from build123d import *

# Parameters (mm, degrees)
SKETCH1_R           = 3
BOSS_EXTRUDE1_DEPTH = 4.3
SKETCH2_R           = 4.92
SKETCH2_R_2         = 3
BOSS_EXTRUDE2_DEPTH = 1.5
FILLET1_R           = 0.6
CHAMFER1_SIZE       = 0.3


with BuildPart() as part:
    # Sketch1 → Boss-Extrude1 (new body)
    with BuildSketch(Plane.XY):
        Polygon((-2.840563324, 4.92), (2.840563324, 4.92), (5.681126649, 0), (2.840563324, -4.92), (-2.840563324, -4.92), (-5.681126649, 0), align=None)
        Circle(SKETCH1_R, mode=Mode.SUBTRACT)
    extrude(amount=BOSS_EXTRUDE1_DEPTH)

    # Sketch2 → Boss-Extrude2 (add)
    with BuildSketch(Plane.XY.offset(4.3)):
        Circle(SKETCH2_R)
        Circle(SKETCH2_R_2, mode=Mode.SUBTRACT)
    extrude(amount=BOSS_EXTRUDE2_DEPTH)

    # Fillet1
    fillet1_edges = [part.edges().sort_by_distance(p)[0] for p in [
        (-4.92, 0, 5.8),
    ]]
    fillet(fillet1_edges, radius=FILLET1_R)

    # Sketch3 → Cut-Revolve1 (revolve, cut)
    with BuildSketch(Plane(origin=(0, 0, 0), x_dir=(0, 0, -1), z_dir=(1, 0, 0))):
        Polygon((-4.3, 4.92), (-3.475971619, 5.575), (-0.824028381, 5.575), (0, 4.92), (0, 6.412884747), (-4.3, 6.412884747), align=None)
    revolve(axis=Axis((0, 0, 0), (0, 0, -1)), mode=Mode.SUBTRACT)

    # Chamfer1
    chamfer1_edges = [part.edges().sort_by_distance(p)[0] for p in [
        (-3, 0, 0),
    ]]
    chamfer(chamfer1_edges, length=CHAMFER1_SIZE)


solid = part.part
The listing builds one solid part. Answer for the finished solid, in the listing's coordinates (mm). Coordinates: 2 decimals unless noted, no trailing zeros. Order: outer loops, then holes, each group sorted by start corner. A loop starts at its lowest first (then second) coordinate and runs counter-clockwise, first axis right, second up.
Q1. A cutting plane is placed at C-C, the plane z = 5.05. Write down the section's boundary in (x, y).
Q2. Given P1, Ø3, axis at x = -0.5, y = 0, coming from the -Z side; P2, Ø3, axis at y = 3, z = 3.5, coming from the -X side, each flat-ended and moving along its own axis, determine where each tip first touches the part or whether it passes through.
Q3. Consider line 1 (Y direction, x = 0, z = 4); line 2 (X direction, y = 1.75, z = 2.65); line 3 (Y direction, x = 2, z = 4.45). Determine where each line is inside the solid, lowest interval first.
Q4. A cutting plane is placed at B-B, the plane z = 1.8. Write down the section's boundary in (x, y) (3 decimals).
Q5. A cutting plane is placed at A-A, the plane y = 0. Write down the section's boundary in (x, z) (3 decimals).
Answers follow:
1. outline: circle Ø9.84 at (0, 0); hole circle Ø6 at (0, 0)
2. P1: passes through
2. P2: stops at x = -4.82
3. line 1: y = -4.92 to -3, 3 to 4.92
3. line 2: x = -4.67 to -2.44, 2.44 to 4.67
3. line 3: y = -4.5 to -2.24, 2.24 to 4.5
4. outline: (-5.572, -0.189) - (-2.95, -4.731) arc R5.575 ccw to (-2.622, -4.92) - (2.622, -4.92) arc R5.575 ccw to (2.95, -4.731) - (5.572, -0.189) arc R5.575 ccw to (5.572, 0.189) - (2.95, 4.731) arc R5.575 ccw to (2.622, 4.92) - (-2.622, 4.92) arc R5.575 ccw to (-2.95, 4.731) - (-5.572, 0.189) arc R5.575 ccw to start; hole circle Ø6 at (0, 0)
5. outline: (-5.575, 0.824) - (-4.92, 0) - (-3.3, 0) - (-3, 0.3) - (-3, 5.8) - (-4.32, 5.8) arc R0.6 ccw to (-4.92, 5.2) - (-4.92, 4.3) - (-5.575, 3.476) - close; (3, 0.3) - (3.3, 0) - (4.92, 0) - (5.575, 0.824) - (5.575, 3.476) - (4.92, 4.3) - (4.92, 5.2) arc R0.6 ccw to (4.32, 5.8) - (3, 5.8) - close
